from build123d import *

# Parameters (mm, degrees)
EXTRUDE_1_DEPTH      = 7.9
EXTRUDE_1_DEPTH_BACK = 7.9
FILLET_1_R           = 0.5


with BuildPart() as part:
    # Эскиз1 → Бобышка-Вытянуть1 (new, two sides: drawn at the far end of the back side and taken through both)
    with BuildSketch(Plane.XY.offset(-EXTRUDE_1_DEPTH_BACK)):
        Polygon((-10.9, 0), (10.9, 0), (10.9, 2.5), (8.4, 2.5), (8.4, 2.3), (2.5, 2.3), (2.5, 2.5), (-2.5, 2.5), (-2.5, 2.3), (-8.4, 2.3), (-8.4, 2.5), (-10.9, 2.5), align=None)
    extrude(amount=EXTRUDE_1_DEPTH + EXTRUDE_1_DEPTH_BACK)

    # Скругление1
    fillet_1_edges = [part.edges().sort_by_distance(p)[0] for p in [
        (8.4, 2.4, -7.9),
        (5.45, 2.3, -7.9),
        (2.5, 2.4, -7.9),
        (-2.5, 2.4, -7.9),
        (-5.45, 2.3, -7.9),
        (-8.4, 2.4, -7.9),
        (10.9, 1.25, 7.9),
        (8.4, 2.4, 7.9),
        (-10.9, 1.25, -7.9),
        (5.45, 2.3, 7.9),
        (2.5, 2.4, 7.9),
        (-2.5, 2.4, 7.9),
        (-5.45, 2.3, 7.9),
        (-8.4, 2.4, 7.9),
        (-10.9, 1.25, 7.9),
        (10.9, 1.25, -7.9),
    ]]
    fillet(fillet_1_edges, radius=FILLET_1_R)


solid = part.part
Input: part model. Units: mm. Frame: model coordinates. A direction names the side the tool comes from. Give positions to 0.01 mm unless a question says otherwise; leave off trailing zeros. Write each loop counter-clockwise with the first axis right and the second up, starting at its lowest first coordinate (ties: lowest second). Pieces come first, ordered by that corner, then holes.
Q1. First-contact query: P1, Ø6.5, axis at x = -5, z = -2.5, coming from the +Y side; P2, Ø1.5, axis at x = 7, z = -5.5, coming from the +Y side. Flat tips, straight axial feed; report the tip coordinate or a pass-through.
Q2. Set-up query: faces 1 (the face through (0, 1, -7.9)), 2 (the face through (5, 2.3, 0)). Return all of +Z, -Z, +X, -X, +Y, -Y with unobstructed straight access to the full face (end or side cutting, diameter ignored); none if empty.
Q3. Material intervals for probe 1 along Y at (x, z) = (5.75, -4), sorted ascending.
Q4. Section A-A, the plane z = -6.5. Output: boundary loops of the cut face in (x, y).
Q5. Section B-B, the plane x = 4. Output: boundary loops of the cut face in (y, z).
Filled in:
1. P1: stops at y = 2.5
1. P2: stops at y = 2.3
2. face 1: -Z, +X, -X, +Y, -Y
2. face 2: +Z, -Z, +Y
3. probe 1: y = 0 to 2.3
4. outline: (-10.9, 0) - (10.9, 0) - (10.9, 2.5) - (8.4, 2.5) - (8.4, 2.3) - (2.5, 2.3) - (2.5, 2.5) - (-2.5, 2.5) - (-2.5, 2.3) - (-8.4, 2.3) - (-8.4, 2.5) - (-10.9, 2.5) - close
5. outline: (0, -7.9) - (1.8, -7.9) arc R0.5 ccw to (2.3, -7.4) - (2.3, 7.4) arc R0.5 ccw to (1.8, 7.9) - (0, 7.9) - close
